Here's how the part is built. I have some questions about the finished solid (model axes, mm). A direction names the side the tool comes from. Give positions to 0.01 mm unless a question says otherwise; leave off trailing zeros. Write each loop counter-clockwise with the first axis right and the second up, starting at its lowest first coordinate (ties: lowest second). Pieces come first, ordered by that corner, then holes. Notation, with made-up numbers: (34.25, -38.5) - (68.25, -38.5) arc R13 cw to (68.25, -16.5) - close; hole circle Ø2 at (0, 33.5). An arc over 180 degrees is marked (long way). One line per item, written item: value. Start each with the question number.
1) Imagine slicing it at A-A on z = -11. Write out the boundary of the cut face in (x, y).
2) Please list where these lines run through material, in increasing order: L1, parallel to Z at x = -0.5, y = 4.5; L2, parallel to Z at x = -1.5, y = 4.5; L3, parallel to Y at x = -1.25, z = -12.5. Write a range as [from, to].
3) On a 3-axis mill with a long thin cutter (end or side, diameter ignored), from which of +Z, -Z, +X, -X, +Y, -Y can I reach the whole of each face in a straight line? I mean faces 1 (the flat face through (-2.7, 3.6, 2.4)), 2 (the cylindrical face through (-1.67, 4.22, -14.79)), 3 (the flat face through (-2.443, 3.278, 1.444)). Say none if no direction works.
4) We'd pull the mould along X, two halves only. Please class faces 4 (the flat face through (-0.675, 3.836, 1.444)), 5 (the flat face through (-0.76, 2.36, 1.44)), 6 (the flat face through (-3, 4, 0)), 7 (the cylindrical face through (1, 3.63, 0.59)): +X half, -X half, draft (parallel to the pull), parting line (faces both ways), or undercut.
5) I'm going to push flat-ended pins straight in: P1, Ø1.5, axis at y = 1.5, z = -4, coming from the +X side; P2, Ø2, axis at x = -1, z = -8.5, coming from the -Y side; P3, Ø2, axis at y = 2, z = -13.5, coming from the -X side. Where does each tip first touch, or does it pass through?
from build123d import *

# Parameters (mm, degrees)
SZKIC1_R                    = 3
DODANIE_WYCI_GNI_CIE2_DEPTH = 2.4
SZKIC2_R                    = 1.5
DODANIE_WYCI_GNI_CIE3_DEPTH = 30
ZAOKR_GLENIE2_R             = 1.2
WYTNIJ_WYCI_GNI_CIE1_DEPTH  = 1.94


with BuildPart() as part:
    # Szkic1 → Dodanie-wyciągnięcie2 (new body)
    with BuildSketch(Plane.XY):
        with Locations((-1.860516246, 2.732142857)):
            Circle(SZKIC1_R)
    extrude(amount=DODANIE_WYCI_GNI_CIE2_DEPTH)

    # Szkic2 → Dodanie-wyciągnięcie3 (add)
    with BuildSketch(Plane(origin=(0, 0, 0), x_dir=(-1, 0, 0), z_dir=(0, 0, -1))):
        with Locations((1.860516246, 2.732142857)):
            Circle(SZKIC2_R)
    extrude(amount=DODANIE_WYCI_GNI_CIE3_DEPTH)

    # Zaokrąglenie2
    zaokr_glenie2_edges = [part.edges().sort_by_distance(p)[0] for p in [
        (-4.860516246, 2.732142857, 2.4),
    ]]
    fillet(zaokr_glenie2_edges, radius=ZAOKR_GLENIE2_R)

    # Szkic3 → Wytnij-wyciągnięcie1 (cut)
    with BuildSketch(Plane.XY.offset(2.4)):
        with BuildLine():
            Line((-1.859548318, 2.959091853), (-0.575649693, 5.316481314))
            ThreePointArc((-0.575649693, 5.316481314), (-0.297886623, 5.158637444), (-0.039271083, 4.97106076))
            Line((-0.039271083, 4.97106076), (-1.329373025, 2.669425378))
            Line((-1.329373025, 2.669425378), (-0.183967515, 2.043621837))
            ThreePointArc((-0.183967515, 2.043621837), (-0.320475658, 1.776553075), (-0.499159616, 1.535654258))
            Line((-0.499159616, 1.535654258), (-1.621312108, 2.148584891))
            Line((-1.621312108, 2.148584891), (-2.819933608, 0.01015725))
            ThreePointArc((-2.819933608, 0.01015725), (-3.083174674, 0.117799023), (-3.33454353, 0.250826496))
            Line((-3.33454353, 0.250826496), (-2.145142944, 2.434706401))
            Line((-2.145142944, 2.434706401), (-3.258687897, 3.042935511))
            ThreePointArc((-3.258687897, 3.042935511), (-3.162842423, 3.328316127), (-3.009463836, 3.587359481))
            Line((-3.009463836, 3.587359481), (-1.859548318, 2.959091853))
        make_face()
    extrude(amount=-WYTNIJ_WYCI_GNI_CIE1_DEPTH, mode=Mode.SUBTRACT)


solid = part.part
Numbers:
1. outline: circle Ø3 at (-1.86, 2.73)
2. L1: [0, 0.46]
2. L2: [0, 2.4]
2. L3: [1.36, 4.1]
3. face 1: +Z, +X, -X, +Y, -Y
3. face 2: -Z
3. face 3: +Z
4. face 4: undercut
4. face 5: undercut
4. face 6: draft
4. face 7: parting line
5. P1: x = -0.44
5. P2: y = 1.23
5. P3: x = -3.36
